from build123d import *

# Parameters (mm, degrees)
F1_DEPTH = 6


with BuildPart() as f1:
    # F0 (on Top) → F1 (new body)
    with BuildSketch(Plane.XY):
        with BuildLine():
            ThreePointArc((-460.478625, -116.977697), (-465.074819, -115.073891), (-466.978625, -110.477697))
            Line((-466.978625, -110.477697), (-466.978625, 81.872303))
            ThreePointArc((-466.978625, 81.872303), (-465.074819, 86.468497), (-460.478625, 88.372303))
            Line((-460.478625, 88.372303), (-243.538855, 88.372303))
            Line((-243.538855, 88.372303), (-107.556077, 88.372303))
            Line((-107.556077, 88.372303), (-107.556077, 89.672303))
            Line((-107.556077, 89.672303), (-442.939144, 89.672303))
            Line((-442.939144, 89.672303), (-460.191501, 89.667017))
            ThreePointArc((-460.191501, 89.667017), (-465.787292, 87.587026), (-468.273338, 82.159427))
            Line((-468.273338, 82.159427), (-468.228486, -111.360677))
            ThreePointArc((-468.228486, -111.360677), (-465.334242, -116.582037), (-459.595644, -118.227558))
            Line((-459.595644, -118.227558), (-3.460598, -118.277697))
            ThreePointArc((-3.460598, -118.277697), (2.054834, -115.99313), (4.339402, -110.477697))
            Line((4.339402, -110.477697), (4.339402, 369.522303))
            ThreePointArc((4.339402, 369.522303), (-3.460598, 377.322303), (-11.260598, 369.522303))
            Line((-11.260598, 369.522303), (-11.260598, 94.554604))
            ThreePointArc((-11.260598, 94.554604), (-13.572677, 91.035911), (-17.556077, 89.672303))
            Line((-17.556077, 89.672303), (-32.556077, 89.672303))
            Line((-32.556077, 89.672303), (-32.556077, 88.372303))
            Line((-32.556077, 88.372303), (-17.556077, 88.372303))
            ThreePointArc((-17.556077, 88.372303), (-11.445398, 91.324664), (-9.960598, 97.946763))
            Line((-9.960598, 97.946763), (-9.960598, 369.522303))
            ThreePointArc((-9.960598, 369.522303), (-3.460598, 376.022303), (3.039402, 369.522303))
            Line((3.039402, 369.522303), (3.039402, -110.477697))
            ThreePointArc((3.039402, -110.477697), (1.135596, -115.073891), (-3.460598, -116.977697))
            Line((-3.460598, -116.977697), (-460.478625, -116.977697))
        make_face()
    extrude(amount=F1_DEPTH)


solid = f1.part
The listing builds one solid part. Answer for the finished solid, in the listing's coordinates (mm). Give positions to 0.01 mm unless a question says otherwise; leave off trailing zeros. Loops run counter-clockwise (first coordinate to the right, second up) from the corner with the lowest first, then second, coordinate; pieces in that order, holes last.
Item 1: Each of these flat-tipped pins is pushed along its axis until it touches: pin 1 Ø1.5 at (y, z) = (287, 5) entering from -X; pin 2 Ø2 at (x, z) = (-355, 5) entering from +Y; pin 3 Ø1.8 at (x, z) = (-24.5, 3) entering from -Y. Where does it stop, or does it pass through?
Derived:
pin 1: stops at x = -11.26
pin 2: stops at y = 89.67
pin 3: stops at y = -118.28
Item 2: A cutting plane is placed at B-B (z = 4.35). Give the vertices of the cut face in (x, y), then the cut area to 3 significant figures.
Derived:
outline: (-468.27, 82.16) - (-468.23, -111.36) arc R7.8 ccw to (-459.6, -118.23) - (-3.46, -118.28) arc R7.8 ccw to (4.34, -110.48) - (4.34, 369.52) arc R7.8 ccw to (-11.26, 369.52) - (-11.26, 94.55) arc R6.5 cw to (-17.56, 89.67) - (-32.56, 89.67) - (-32.56, 88.37) - (-17.56, 88.37) arc R7.8 ccw to (-9.96, 97.95) - (-9.96, 369.52) arc R6.5 cw to (3.04, 369.52) - (3.04, -110.48) arc R6.5 cw to (-3.46, -116.98) - (-460.48, -116.98) arc R6.5 cw to (-466.98, -110.48) - (-466.98, 81.87) arc R6.5 cw to (-460.48, 88.37) - (-107.56, 88.37) - (-107.56, 89.67) - (-442.94, 89.67) - (-460.19, 89.67) arc R7.8 ccw to start
area: 2,370 mm2
Item 3: A cutting plane is placed at D-D (x = -96.5). Give the vertices of the cut face in (y, z), then the cut area to 3 significant figures.
Derived:
outline: (-118.27, 0) - (-116.98, 0) - (-116.98, 6) - (-118.27, 6) - close
area: 7.74 mm2
Item 4: A cutting plane is placed at A-A (y = 197.5). Give the vertices of the cut face in (x, z), then the cut area to 3 significant figures.
Derived:
outline: (-11.26, 0) - (-9.96, 0) - (-9.96, 6) - (-11.26, 6) - close; (3.04, 0) - (4.34, 0) - (4.34, 6) - (3.04, 6) - close
area: 15.6 mm2
Item 5: A cutting plane is placed at C-C (x = -409). Give the vertices of the cut face in (y, z), then the cut area to 3 significant figures.
Derived:
outline: (-118.23, 0) - (-116.98, 0) - (-116.98, 6) - (-118.23, 6) - close; (88.37, 0) - (89.67, 0) - (89.67, 6) - (88.37, 6) - close
area: 15.3 mm2
Item 6: Find the intervals of material crossed by line 1 along Y through (x, z) = (-161.5, 0.85); line 2 along X through (y, z) = (284.5, 4.8); line 3 along X through (y, z) = (-93.5, 2.5), in increasing order.
Derived:
line 1: y = -118.26 to -116.98, 88.37 to 89.67
line 2: x = -11.26 to -9.96, 3.04 to 4.34
line 3: x = -468.23 to -466.98, 3.04 to 4.34
